```python
from build123d import *

# Parameters (mm, degrees)
F0_R     = 35
F0_R_2   = 2.5
F0_R_3   = 25
F1_DEPTH = 25
F0_R_4   = 15
F2_DEPTH = 55


# Not quite as in the source:
# - the program builds the solid bodies; features that only make, move or delete a surface that nothing else refers to are left out


with BuildPart() as f1:
    # F0 (on Top) → F1 (new body)
    with BuildSketch(Plane.XY):
        Circle(F0_R)
        with Locations((-22.9813332936, -19.2836282906)):
            Circle(F0_R_2, mode=Mode.SUBTRACT)
        with Locations((22.9813332936, -19.2836282906)):
            Circle(F0_R_2, mode=Mode.SUBTRACT)
        Circle(F0_R_3, mode=Mode.SUBTRACT)
        with Locations((0, 30)):
            Circle(F0_R_2, mode=Mode.SUBTRACT)
    extrude(amount=F1_DEPTH)

    # F0 (on Top) → F2 (join)
    with BuildSketch(Plane.XY):
        Circle(F0_R_3)
        Circle(F0_R_4, mode=Mode.SUBTRACT)
    extrude(amount=F2_DEPTH)


solid = f1.part
```
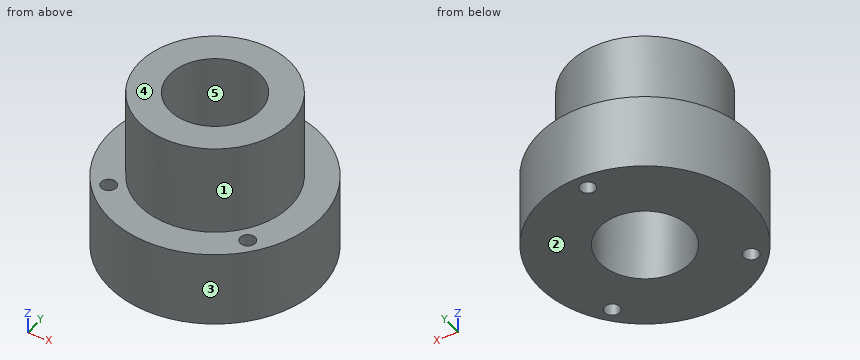
Verification items for the finished model (mm, model axes). Face numbers are marked on the shaded views. A direction names the side the tool comes from. Coordinates: 2 decimals unless noted, no trailing zeros. Write each loop counter-clockwise with the first axis right and the second up, starting at its lowest first coordinate (ties: lowest second). Pieces come first, ordered by that corner, then holes. Notation, with made-up numbers: M 47,3 L 104,3 A30 ccw 104,35 Z; hole C -20,48 d6. An arc over 180 degrees is marked long. Answer as a JSON object with one key per item and string values. Group by question number.
(1) Cross-section at D-D, the plane z = 12. Record the cut outline in (x, y), and give its area (3 significant figures).
(2) Material ranges on line 1 (Y direction, x = 0, z = 5.5); line 2 (Y direction, x = 0.5, z = 27.5) (3 decimals); line 3 (Z direction, x = -31.5, y = -3), recorded low to high.
(3) Cross-section at A-A, the plane y = 0. Record the cut outline in (x, z), and give its area (3 significant figures).
(4) Release check for a two-part mould opening along X. For the marked faces 3, 4 and 5 record: +X half, -X half, draft (parallel to the pull), parting line (faces both ways), or undercut.
(5) Cross-section at C-C, the plane x = 23.5. Record the cut outline in (y, z), and give its area (3 significant figures).
(6) Cross-section at B-B, the plane x = 0. Record the cut outline in (y, z), and give its area (4 significant figures).
(7) Tool access check on the marked faces 1 and 2. Record the directions out of +Z, -Z, +X, -X, +Y, -Y that give a thin tool (end or side, any length) a straight path to the whole face; none if there is none.
(8) Gauge pin test, flat ends, axial feed: pin 1 (2 mm diameter, centred on y = 23, z = 40, fed in from -X); pin 2 (8 mm diameter, centred on y = -27, z = 35.5, fed in from -X); pin 3 (1.5 mm diameter, centred on x = -18.5, z = 17.5, fed in from -Y); pin 4 (4.5 mm diameter, centred on x = 22.98, y = -19.28, fed in from +Z) (1 decimal). Record the tip position at first contact, or that the pin passes through.
Reply:
{
 "1": {"outline": "C 0,0 d70; hole C -22.98,-19.28 d5; hole C 0,0 d30; hole C 0,30 d5; hole C 22.98,-19.28 d5", "area": "3,080 mm²"},
 "2": {"line 1": "-35 to -15, 15 to 27.5, 32.5 to 35", "line 2": "-24.995 to -14.992, 14.992 to 24.995", "line 3": "0 to 25"},
 "3": {"outline": "M -35,0 L -15,0 L -15,55 L -25,55 L -25,25 L -35,25 Z; M 15,0 L 35,0 L 35,25 L 25,25 L 25,55 L 15,55 Z", "area": "1,600 mm²"},
 "4": {"face 3": "parting line", "face 4": "draft", "face 5": "undercut"},
 "5": {"outline": "M -25.94,0 L -21.73,0 L -21.73,25 L -25.94,25 Z; M -16.84,0 L 25.94,0 L 25.94,25 L 8.53,25 L 8.53,55 L -8.53,55 L -8.53,25 L -16.84,25 Z", "area": "1,690 mm²"},
 "6": {"outline": "M -35,0 L -15,0 L -15,55 L -25,55 L -25,25 L -35,25 Z; M 15,0 L 27.5,0 L 27.5,25 L 25,25 L 25,55 L 15,55 Z; M 32.5,0 L 35,0 L 35,25 L 32.5,25 Z", "area": "1,475 mm²"},
 "7": {"face 1": "+Z", "face 2": "-Z, +X, -X, +Y, -Y"},
 "8": {"pin 1": "x = -11.87", "pin 2": "x = -9.8", "pin 3": "y = -30.17", "pin 4": "through"}
}
